from build123d import *

# Parameters (mm, degrees)
PLATE_DEPTH             = 9
SKETCH3_R               = 1.6
HEX_HOLES_DEPTH         = 128.597021909
SKETCH4_W               = 20
SKETCH4_H               = 5
BATTERY_HOLDER_DEPTH    = 20
SKETCH5_W               = 42
SKETCH5_H               = 42
SKETCH5_R               = 12
SKETCH5_R_2             = 1.55
BOSS_EXTRUDE2_DEPTH     = 5
BOSS_EXTRUDE3_START     = -5
SKETCH6_W               = 42
SKETCH6_H               = 42
SKETCH6_R               = 12
SKETCH6_R_2             = 1.55
BOSS_EXTRUDE3_DEPTH     = 5
SKETCH8_R               = 14.25
BOSS_EXTRUDE4_DEPTH     = 12
SKETCH7_R               = 11.75
CUT_EXTRUDE1_DEPTH      = 10.6
CASTER_HOLES_DEPTH      = 135.029847422
CASTER_HOLES_DEPTH_BACK = 135.029847422
SKETCH2_R               = 1.09


with BuildPart() as part:
    # Sketch1 → Plate (new body)
    with BuildSketch(Plane(origin=(0, 0, 0), x_dir=(1, 0, 0), z_dir=(0, 1, 0))):
        with BuildLine():
            Line((-65, -90), (65, -90))
            ThreePointArc((65, -90), (82.67766953, -82.67766953), (90, -65))
            Line((90, -65), (90, 65))
            ThreePointArc((90, 65), (82.67766953, 82.67766953), (65, 90))
            Line((65, 90), (-65, 90))
            ThreePointArc((-65, 90), (-82.67766953, 82.67766953), (-90, 65))
            Line((-90, 65), (-90, -65))
            ThreePointArc((-90, -65), (-82.67766953, -82.67766953), (-65, -90))
        make_face()
    extrude(amount=PLATE_DEPTH)

    # Sketch3 → Hex Holes (cut, through all)
    with BuildSketch(Plane(origin=(0, 9, 0), x_dir=(1, 0, 0), z_dir=(0, 1, 0))):
        with Locations(Location((-65, 80, 0), (0, 0, 270))):
            Circle(SKETCH3_R)
        with Locations(Location((-80, 65, 0), (0, 0, 270))):
            Circle(SKETCH3_R)
        with Locations(Location((80, 65, 0), (0, 0, 270))):
            Circle(SKETCH3_R)
        with Locations(Location((80, -65, 0), (0, 0, 270))):
            Circle(SKETCH3_R)
        with Locations(Location((65, 80, 0), (0, 0, 270))):
            Circle(SKETCH3_R)
        with Locations(Location((65, -80, 0), (0, 0, 270))):
            Circle(SKETCH3_R)
        with Locations(Location((-65, -80, 0), (0, 0, 270))):
            Circle(SKETCH3_R)
        with Locations(Location((-80, -65, 0), (0, 0, 270))):
            Circle(SKETCH3_R)
    extrude(amount=-HEX_HOLES_DEPTH, mode=Mode.SUBTRACT)

    # Sketch4 → Battery Holder (add)
    with BuildSketch(Plane(origin=(0, 9, 0), x_dir=(1, 0, 0), z_dir=(0, 1, 0))):
        Polygon((-22, -85), (-17, -85), (-17, -90), (-27, -90), (-27, -80), (-22, -80), align=None)
        Polygon((17, -85), (22, -85), (22, -80), (27, -80), (27, -90), (17, -90), align=None)
        with Locations((0, 56)):
            Rectangle(SKETCH4_W, SKETCH4_H)
    extrude(amount=BATTERY_HOLDER_DEPTH)

    # Sketch5 → Boss-Extrude2 (add)
    with BuildSketch(Plane.ZY.offset(90)):
        with Locations((29, 30)):
            Rectangle(SKETCH5_W, SKETCH5_H)
        with Locations((29, 30)):
            Circle(SKETCH5_R, mode=Mode.SUBTRACT)
        with Locations((13.5, 45.5)):
            Circle(SKETCH5_R_2, mode=Mode.SUBTRACT)
        with Locations((44.5, 45.5)):
            Circle(SKETCH5_R_2, mode=Mode.SUBTRACT)
        with Locations((44.5, 14.5)):
            Circle(SKETCH5_R_2, mode=Mode.SUBTRACT)
        with Locations((13.5, 14.5)):
            Circle(SKETCH5_R_2, mode=Mode.SUBTRACT)
    extrude(amount=-BOSS_EXTRUDE2_DEPTH)

    # Sketch6 → Boss-Extrude3 (add)
    with BuildSketch(Plane(origin=(90, 0, 0), x_dir=(0, 0, -1), z_dir=(1, 0, 0)).offset(BOSS_EXTRUDE3_START)):
        with Locations((-29, 30)):
            Rectangle(SKETCH6_W, SKETCH6_H)
        with Locations(Location((-29, 30, 0), (0, 0, 180))):
            Circle(SKETCH6_R, mode=Mode.SUBTRACT)
        with Locations(Location((-44.5, 45.5, 0), (0, 0, 180))):
            Circle(SKETCH6_R_2, mode=Mode.SUBTRACT)
        with Locations(Location((-13.5, 45.5, 0), (0, 0, 180))):
            Circle(SKETCH6_R_2, mode=Mode.SUBTRACT)
        with Locations(Location((-13.5, 14.5, 0), (0, 0, 180))):
            Circle(SKETCH6_R_2, mode=Mode.SUBTRACT)
        with Locations(Location((-44.5, 14.5, 0), (0, 0, 180))):
            Circle(SKETCH6_R_2, mode=Mode.SUBTRACT)
    extrude(amount=BOSS_EXTRUDE3_DEPTH)

    # Sketch8 → Boss-Extrude4 (add)
    with BuildSketch(Plane(origin=(0, 9, 0), x_dir=(1, 0, 0), z_dir=(0, 1, 0))):
        with Locations((0, 70)):
            Circle(SKETCH8_R)
    extrude(amount=BOSS_EXTRUDE4_DEPTH)

    # Sketch7 → Cut-Extrude1 (cut)
    with BuildSketch(Plane.XZ):
        with Locations(Location((0, -70, 0), (0, 0, 270))):
            Circle(SKETCH7_R)
    extrude(amount=-CUT_EXTRUDE1_DEPTH, mode=Mode.SUBTRACT)

    # Sketch2 → Caster Holes (cut, two sides: drawn at the far end of the back side and taken through both)
    with BuildSketch(Plane(origin=(0, 9, 0), x_dir=(1, 0, 0), z_dir=(0, 1, 0)).offset(-CASTER_HOLES_DEPTH_BACK)):
        with Locations(Location((-7.747, 70, 0), (0, 0, 270))):
            Circle(SKETCH2_R)
        with Locations(Location((7.747, 70, 0), (0, 0, 270))):
            Circle(SKETCH2_R)
    extrude(amount=CASTER_HOLES_DEPTH + CASTER_HOLES_DEPTH_BACK, mode=Mode.SUBTRACT)


solid = part.part
Here's how the part is built. I have some questions about the finished solid (model axes, mm). A direction names the side the tool comes from. Round coordinates to 2 decimals unless told otherwise and drop trailing zeros. Order: outer loops, then holes, each group sorted by start corner. A loop starts at its lowest first (then second) coordinate and runs counter-clockwise, first axis right, second up. Notation, with made-up numbers: M -32,78.5 L 5,78.5 A20 ccw 5,110.5 Z; hole C 1.25,35.5 d9. An arc over 180 degrees is marked long. Return JSON: item names as keys, results as strings. Group by question number.
1. I'm going to push flat-ended pins straight in: pin 1 Ø1.5 at (y, z) = (18.5, 83) entering from +X; pin 2 Ø2 at (x, z) = (-58.5, -40.5) entering from +Y; pin 3 Ø10 at (x, y) = (4, 19) entering from -Z. Where does each tip first touch, or does it pass through?
2. If we section it at A-A on x = 0: List the corners of the cut face in (y, z) for me.
3. On a 3-axis mill with a long thin cutter (end or side, diameter ignored), from which of +Z, -Z, +X, -X, +Y, -Y can I reach the whole of each face in a straight line? I mean faces 1 (the face through (-88, 30, 50)), 2 (the face through (10, 19, -56)), 3 (the face through (3.529, 5.226, -81.207)), 4 (the face through (19, 19, 85)). Say none if no direction works.
4. If we section it at D-D on x = -38: List the corners of the cut face in (y, z) for me, then the cut area to 3 significant figures.
5. If we section it at B-B on y = 25.5: State how many separate pieces and enclosed holes the cut face has, then the cut area to 3 significant figures.
6. If we mould it in two halves opening along Y, with no side actions, what happens to faces 5 (the face through (24, 19, 80)), 6 (the face through (87.465, 26.396, 40.446)), 7 (the face through (0, 10.6, -70))? For each: pulls with the +Y half, pulls with the -Y half, needs draft (parallel to the pull), parting line crosses it, or undercut.
7. If we section it at C-C on z = 55.5: List the corners of the cut face in (x, y) for me.
8. Please list where these lines run through material, in increasing order: probe 1 along Z at (x, y) = (86.3, 14.5); probe 2 along Y at (x, z) = (86.2, 13.5); probe 3 along X at (y, z) = (13.5, -70).
Reply:
{
 "1": {"pin 1": "x = 27", "pin 2": "y = 9", "pin 3": "z = -84.25"},
 "2": {"outline": "M 0,-90 L 9,-90 L 9,-84.25 L 21,-84.25 L 21,-58.5 L 29,-58.5 L 29,-53.5 L 9,-53.5 L 9,90 L 0,90 L 0,-58.25 L 10.6,-58.25 L 10.6,-81.75 L 0,-81.75 Z"},
 "3": {"face 1": "+Z, +X, -X, +Y", "face 2": "+Z, +X, +Y", "face 3": "-Y", "face 4": "-Z, +Y"},
 "4": {"outline": "M 0,-90 L 9,-90 L 9,90 L 0,90 Z", "area": "1,620 mm^2"},
 "5": {"separate pieces": "7", "enclosed holes": "0", "area": "448 mm^2"},
 "6": {"face 5": "needs draft", "face 6": "undercut", "face 7": "pulls with the -Y half"},
 "7": {"outline": "M -90,0 L 90,0 L 90,9 L -90,9 Z"},
 "8": {"probe 1": "8 to 11.95, 15.05 to 42.95, 46.05 to 50", "probe 2": "0 to 12.95, 16.05 to 43.95, 47.05 to 51", "probe 3": "-14.25 to -8.84, -6.66 to 6.66, 8.84 to 14.25"}
}
